from build123d import *

# Parameters (mm, degrees)
BOSS_EXTRUDE1_DEPTH = 80
SKETCH2_R           = 2.5
CUT_EXTRUDE1_DEPTH  = 107.77078252
SKETCH3_R           = 2.5
CUT_EXTRUDE2_DEPTH  = 107.77078252


with BuildPart() as part:
    # Sketch1 → Boss-Extrude1 (new, symmetric)
    with BuildSketch(Plane(origin=(0, 0, 0), x_dir=(1, 0, 0), z_dir=(0, 1, 0))):
        Polygon((0, 0), (0, 50), (5, 50), (5, 5), (50, 5), (50, 0), align=None)
    extrude(amount=BOSS_EXTRUDE1_DEPTH, both=True)

    # Sketch2 → Cut-Extrude1 (cut, through all)
    with BuildSketch(Plane.XY):
        with Locations((25, 55)):
            Circle(SKETCH2_R)
        with Locations((25, -55)):
            Circle(SKETCH2_R)
    extrude(amount=-CUT_EXTRUDE1_DEPTH, mode=Mode.SUBTRACT)

    # Sketch3 → Cut-Extrude2 (cut, through all)
    with BuildSketch(Plane.ZY):
        with Locations((-25, 55)):
            Circle(SKETCH3_R)
        with Locations((-25, -55)):
            Circle(SKETCH3_R)
    extrude(amount=-CUT_EXTRUDE2_DEPTH, mode=Mode.SUBTRACT)


solid = part.part
Input: part model. Units: mm. Frame: model coordinates. A direction names the side the tool comes from. Coordinates: 2 decimals unless noted, no trailing zeros. Order: outer loops, then holes, each group sorted by start corner. A loop starts at its lowest first (then second) coordinate and runs counter-clockwise, first axis right, second up. Notation, with made-up numbers: M 35.25,32 L 70.25,32 A19 cw 70.25,43 Z; hole C -40,83.5 d5. An arc over 180 degrees is marked long. Write item = value, one per line. Start each with the question number.
(1) Pull-direction query (Y, two-part tool) for faces 1 (the flat face through (5, 1, -28)), 2 (the cylindrical face through (2.46, -53.31, -26.84)), 3 (the flat face through (14, 80, -4.7)); classes: released by +Y, released by -Y, zero draft, split by the parting line, or undercut.
(2) Section C-C on y = -55. Output: boundary loops of the cut face in (x, z), and give its area (3 significant figures).
(3) Section B-B on x = 25. Output: boundary loops of the cut face in (y, z).
(4) Section D-D on y = 40.5. Output: boundary loops of the cut face in (x, z), and give its area (3 significant figures).
(5) Section A-A on z = -25. Output: boundary loops of the cut face in (x, y).
(6) Line query: line 1 along Y through (x, z) = (3, -25); line 2 along X through (y, z) = (65, -10.5); line 3 along Z through (x, y) = (11, 16.5). Output: solid intervals per line, ascending. Write a range as [from, to].
(7) First-contact query: P1, Ø8, axis at y = -55, z = -25, coming from the +X side; P2, Ø22.5, axis at x = 35.5, y = 38.5, coming from the -Z side. Flat tips, straight axial feed; report the tip coordinate or a pass-through.
(8) Reachability of faces 4 (the flat face through (25, 1, 0)), 5 (the flat face through (27, 1, -5)) from +Z, -Z, +X, -X, +Y, -Y: full face, straight path, thin tool, end or side. Return the list, or none.
Result set:
q1.face_1 = zero draft
q1.face_2 = undercut
q1.face_3 = released by +Y
q2.outline = M 0,-50 L 5,-50 L 5,-27.5 L 0,-27.5 Z; M 0,-22.5 L 5,-22.5 L 5,-5 L 22.5,-5 L 22.5,0 L 0,0 Z; M 27.5,-5 L 50,-5 L 50,0 L 27.5,0 Z
q2.area = 425 mm²
q3.outline = M -80,-5 L -57.5,-5 L -57.5,0 L -80,0 Z; M -52.5,-5 L 52.5,-5 L 52.5,0 L -52.5,0 Z; M 57.5,-5 L 80,-5 L 80,0 L 57.5,0 Z
q4.outline = M 0,-50 L 5,-50 L 5,-5 L 50,-5 L 50,0 L 0,0 Z
q4.area = 475 mm²
q5.outline = M 0,-80 L 5,-80 L 5,-57.5 L 0,-57.5 Z; M 0,-52.5 L 5,-52.5 L 5,52.5 L 0,52.5 Z; M 0,57.5 L 5,57.5 L 5,80 L 0,80 Z
q6.line_1 = [-80, -57.5], [-52.5, 52.5], [57.5, 80]
q6.line_2 = [0, 5]
q6.line_3 = [-5, 0]
q7.P1 = 5
q7.P2 = -5
q8.face_4 = +Z, +X, -X, +Y, -Y
q8.face_5 = -Z, +X, +Y, -Y
